Verification items for the finished model (mm, model axes). Give positions to 0.01 mm unless a question says otherwise; leave off trailing zeros. Loops run counter-clockwise (first coordinate to the right, second up) from the corner with the lowest first, then second, coordinate; pieces in that order, holes last. Notation, with made-up numbers: (-14, -36) - (7, -36) arc R10 ccw to (7, -18) - close; hole circle Ø2 at (33.25, 87.25). An arc over 180 degrees is marked (long way). One line per question, with ' | ' between items. Start each with the question number.
1. Depth check by flat-ended pin: pin 1 Ø3.5 at (x, y) = (0, -12.7) entering from -Z; pin 2 Ø1.6 at (x, z) = (34, 1) entering from +Y. Enter the tip coordinate at first touch or a pass-through.
2. Section check C-C, the plane y = -19. Enter the section's corners in (x, z) (3 decimals), then the cut area to 3 significant figures.
3. Section check A-A, the plane x = 38.1. Enter the section's corners in (y, z) (3 decimals).
4. Section check D-D, the plane z = 2.5. State how many separate pieces and enclosed holes the cut face has, then the cut area to 3 significant figures.
5. Section check B-B, the plane y = 0. Enter the section's corners in (x, z) (3 decimals), then the cut area to 3 significant figures.
6. Thickness scan on line 1 along X through (y, z) = (-25.5, 0.6); line 2 along Y through (x, z) = (-52, 0.95) (3 decimals); line 3 along Y through (x, z) = (38.1, 1.2). Record the ranges inside material, lowest first. Write a range as from..to.
from build123d import *

# Parameters (mm, degrees)
SKETCH1_R           = 2.032
SKETCH1_R_2         = 14.351
SKETCH1_W           = 25.4
SKETCH1_H           = 76.2
BOSS_EXTRUDE1_DEPTH = 3.175
SKETCH2_R           = 2.032
CUT_EXTRUDE1_DEPTH  = 69.759094853
SKETCH4_W           = 3.175
SKETCH4_H           = 25.4
BOSS_EXTRUDE2_DEPTH = 38.1
SKETCH5_R           = 2.032
CUT_EXTRUDE2_DEPTH  = 69.759094853
FILLET5_R           = 2.54
SKETCH6_W           = 12.7
SKETCH6_H           = 12.7
SKETCH6_R           = 2.159
BOSS_EXTRUDE3_DEPTH = 3.175
FILLET6_R           = 2.54


with BuildPart() as part:
    # Sketch1 → Boss-Extrude1 (new body)
    # profile 1 of 2: a face of its own
    with BuildSketch(Plane.XY):
        Polygon((-57.15, -34.095), (-12.7, -34.095), (-12.7, -24.638), (-12.7, 12.895), (-57.15, 12.895), align=None)
        with Locations((-52.959, -28.634)):
            Circle(SKETCH1_R, mode=Mode.SUBTRACT)
        with Locations((-34.925, -10.6)):
            Circle(SKETCH1_R_2, mode=Mode.SUBTRACT)
        with Locations((-16.891, -28.634)):
            Circle(SKETCH1_R, mode=Mode.SUBTRACT)
        with Locations((-52.959, 7.434)):
            Circle(SKETCH1_R, mode=Mode.SUBTRACT)
    # profile 2 of 2: a face of its own
    with BuildSketch(Plane.XY):
        Rectangle(SKETCH1_W, SKETCH1_H)
    extrude(amount=BOSS_EXTRUDE1_DEPTH)

    # Sketch2 → Cut-Extrude1 (cut, through all)
    with BuildSketch(Plane.XY.offset(3.175)):
        Circle(SKETCH2_R)
        with Locations((0, 12.7)):
            Circle(SKETCH2_R)
        with Locations((0, 25.4)):
            Circle(SKETCH2_R)
        with Locations((0, -12.7)):
            Circle(SKETCH2_R)
        with Locations((0, -25.4)):
            Circle(SKETCH2_R)
    extrude(amount=-CUT_EXTRUDE1_DEPTH, mode=Mode.SUBTRACT)

    # Sketch4 → Boss-Extrude2 (add)
    with BuildSketch(Plane(origin=(12.7, 0, 0), x_dir=(0, 0, -1), z_dir=(1, 0, 0))):
        with Locations((-1.5875, -25.4)):
            Rectangle(SKETCH4_W, SKETCH4_H)
    extrude(amount=BOSS_EXTRUDE2_DEPTH)

    # Sketch5 → Cut-Extrude2 (cut, through all)
    with BuildSketch(Plane(origin=(0, 0, 0), x_dir=(-1, 0, 0), z_dir=(0, 0, -1))):
        with Locations(Location((0, -25.4, 0), (0, 0, 180))):
            Circle(SKETCH5_R)
        with Locations((-12.7, -25.4)):
            Circle(SKETCH5_R)
        with Locations((-25.4, -25.4)):
            Circle(SKETCH5_R)
        with Locations((-38.1, -25.4)):
            Circle(SKETCH5_R)
    extrude(amount=-CUT_EXTRUDE2_DEPTH, mode=Mode.SUBTRACT)

    # Fillet5
    fillet5_edges = [part.edges().sort_by_distance(p)[0] for p in [
        (-12.7, -38.1, 1.5875),
        (-57.15, -34.095, 1.5875),
        (-57.15, 12.895, 1.5875),
        (-12.7, 12.895, 1.5875),
        (-12.7, 38.1, 1.5875),
        (12.7, 38.1, 1.5875),
        (12.7, -12.7, 1.5875),
        (50.8, -38.1, 1.5875),
        (50.8, -12.7, 1.5875),
    ]]
    fillet(fillet5_edges, radius=FILLET5_R)

    # Sketch6 → Boss-Extrude3 (add)
    with BuildSketch(Plane.XY.offset(3.175)):
        with Locations((-19.05, 19.245)):
            Rectangle(SKETCH6_W, SKETCH6_H)
        with Locations((-19.05, 19.245)):
            Circle(SKETCH6_R, mode=Mode.SUBTRACT)
    extrude(amount=-BOSS_EXTRUDE3_DEPTH)

    # Fillet6
    fillet6_edges = [part.edges().sort_by_distance(p)[0] for p in [
        (-25.4, 25.595, 1.5875),
    ]]
    fillet(fillet6_edges, radius=FILLET6_R)


solid = part.part
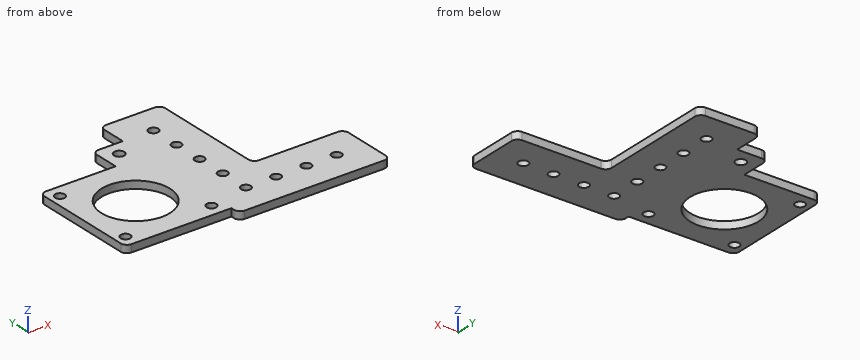
Results list:
1) pin 1: through | pin 2: y = -12.7
2) outline: (-57.15, 0) - (-46.561, 0) - (-46.561, 3.175) - (-57.15, 3.175) - close; (-23.289, 0) - (50.8, 0) - (50.8, 3.175) - (-23.289, 3.175) - close | area: 269 mm²
3) outline: (-38.1, 0) - (-27.432, 0) - (-27.432, 3.175) - (-38.1, 3.175) - close; (-23.368, 0) - (-12.7, 0) - (-12.7, 3.175) - (-23.368, 3.175) - close
4) separate pieces: 1 | enclosed holes: 13 | area: 4,340 mm²
5) outline: (-57.15, 0) - (-44.599, 0) - (-44.599, 3.175) - (-57.15, 3.175) - close; (-25.251, 0) - (-2.032, 0) - (-2.032, 3.175) - (-25.251, 3.175) - close; (2.032, 0) - (12.7, 0) - (12.7, 3.175) - (2.032, 3.175) - close | area: 147 mm²
6) line 1: -57.15..-2.03, 2.03..10.67, 14.73..23.37, 27.43..36.07, 40.13..50.8 | line 2: -34.095..-30.425, -26.843..5.643, 9.225..12.895 | line 3: -38.1..-27.43, -23.37..-12.7
